from build123d import *

# Parameters (mm, degrees)
SKETCH_1_W      = 7.4
SKETCH_1_H      = 7.1
SKETCH_1_R      = 1.75
EXTRUDE_1_DEPTH = 6.4
SKETCH_1_3_R    = 1.75
EXTRUDE_2_DEPTH = 1.3
CHAMFER_1_SIZE  = 5
CHAMFER_1_SIZE2 = 2.331538291


with BuildPart() as part:
    # Sketch 1 → Extrude 1 (new body)
    # profile 1 of 2: a face of its own
    with BuildSketch(Plane.XY):
        with Locations((-2.9453125, -2.68046875)):
            Rectangle(SKETCH_1_W, SKETCH_1_H)
        with Locations((-2.9453125, -2.38046875)):
            Circle(SKETCH_1_R, mode=Mode.SUBTRACT)
    # profile 2 of 2: a face of its own
    with BuildSketch(Plane.XY):
        with Locations((-2.9453125, -2.38046875)):
            Circle(SKETCH_1_R)
    extrude(amount=EXTRUDE_1_DEPTH)

    # Sketch 1_3 → Extrude 2 (add)
    with BuildSketch(Plane.XY):
        with Locations((-2.9453125, -2.38046875)):
            Circle(SKETCH_1_3_R)
    extrude(amount=-EXTRUDE_2_DEPTH)

    # Chamfer 1
    chamfer_1_edges = [part.edges().sort_by_distance(p)[0] for p in [
        (-2.9453125, 0.86953125, 6.4),
    ]]
    chamfer_1_side = [part.faces().sort_by_distance(p)[0] for p in [
        (-2.9453125, -2.68046875, 6.4),
    ]]
    chamfer(chamfer_1_edges, length=CHAMFER_1_SIZE, length2=CHAMFER_1_SIZE2, reference=chamfer_1_side[0])


solid = part.part
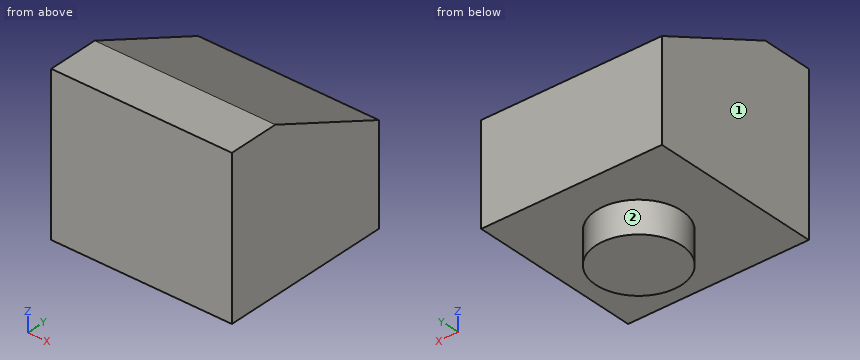
Can you work these out from the model? Positions are in its coordinate system, mm. Face numbers are marked on the shaded views. A direction names the side the tool comes from. Give positions to 0.01 mm unless a question says otherwise; leave off trailing zeros. Write each loop counter-clockwise with the first axis right and the second up, starting at its lowest first coordinate (ties: lowest second). Pieces come first, ordered by that corner, then holes. Notation, with made-up numbers: (7.25, 35.25) -> (45.25, 35.25) arc R15 ccw to (45.25, 41.25) -> close; hole circle Ø8 at (31.5, -0.5). An arc over 180 degrees is marked (long way). Answer as a JSON object with one key per item and string values. Group by question number.
Item 1: Suppose I cut it at A-A (x = -2.25). Please give me the cut outline in (y, z), plus the area to 3 significant figures.
Item 2: Suppose I cut it at B-B (y = -3.5). Please give me the cut outline in (x, z).
Item 3: Suppose I cut it at D-D (x = -6). Please give me the cut outline in (y, z).
Item 4: I'm going to push a flat-ended pin straight in: P1, Ø2, axis at x = -5.5, y = -0.5, coming from the -Z side. Where does the tip first touch, or does it pass through?
Item 5: Suppose I cut it at C-C (z = -0.5). Please give me the cut outline in (x, y), plus the area to 3 significant figures.
Item 6: Please list where these lines run through material, in increasing order: line 1 (Z direction, x = -5, y = -4.75); line 2 (Z direction, x = 0, y = -2.5); line 3 (Y direction, x = -5.5, z = 5.25). Write a range as [from, to].
Item 7: For the marked faces 1 and 2, which set-ups out of +Z, -Z, +X, -X, +Y, -Y let a thin tool reach every point of the face, with its end or its side?
Findings:
{
 "1": {"outline": "(-6.23, 0) -> (-3.99, 0) -> (-3.99, -1.3) -> (-0.77, -1.3) -> (-0.77, 0) -> (0.87, 0) -> (0.87, 4.07) -> (-4.13, 6.4) -> (-6.23, 6.4) -> close", "area": "43.8 mm²"},
 "2": {"outline": "(-6.65, 0) -> (-4.29, 0) -> (-4.29, -1.3) -> (-1.6, -1.3) -> (-1.6, 0) -> (0.75, 0) -> (0.75, 6.11) -> (-6.65, 6.11) -> close"},
 "3": {"outline": "(-6.23, 0) -> (0.87, 0) -> (0.87, 4.07) -> (-4.13, 6.4) -> (-6.23, 6.4) -> close"},
 "4": {"P1": "stops at z = 0"},
 "5": {"outline": "circle Ø3.5 at (-2.95, -2.38)", "area": "9.62 mm²"},
 "6": {"line 1": "z = [0, 6.4]", "line 2": "z = [0, 5.64]", "line 3": "y = [-6.23, -1.66]"},
 "7": {"face 1": "+Z, -Z, -X, +Y, -Y", "face 2": "-Z"}
}
